Geometry check sheet. Reference: drawing and pictorial views, mm from the part's lowest x, y, z. A direction names the side the tool comes from. Coordinates: 2 decimals unless noted, no trailing zeros. Write each loop counter-clockwise with the first axis right and the second up, starting at its lowest first coordinate (ties: lowest second). Pieces come first, ordered by that corner, then holes. Notation, with made-up numbers: M 48.25,55 L 83.25,55 A23 ccw 83.25,91 Z; hole C 74.5,53 d7. An arc over 180 degrees is marked long. One line per item, written item: value.
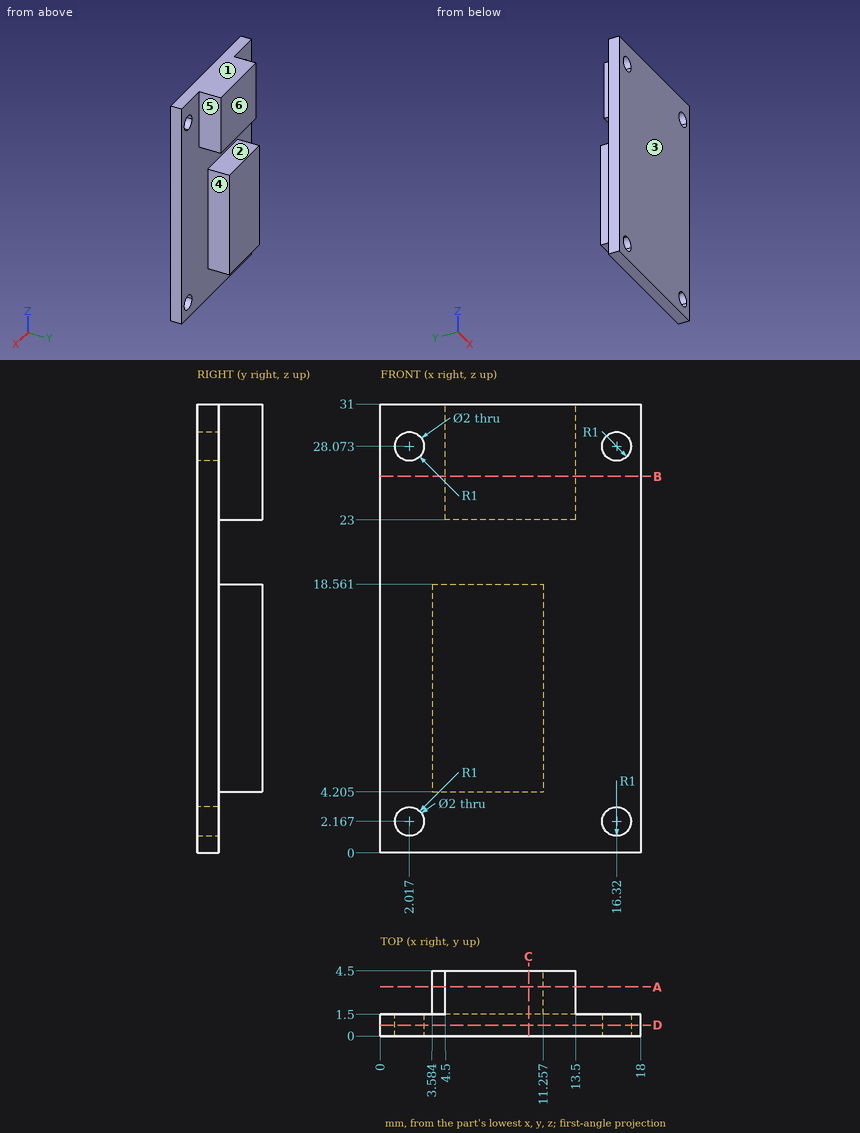
Item 1: Scan lines: line 1 (Z direction, x = 9.25, y = 4.15) (1 decimal); line 2 (Z direction, x = 12.5, y = 2.8); line 3 (Y direction, x = 5.25, z = 3). Record each from-to range of solid material in increasing order.
The answers:
line 1: z = 4.2 to 18.6, 23 to 31
line 2: z = 23 to 31
line 3: y = 0 to 1.5
Item 2: Cross-section at D-D, the plane y = 0.75. Enter the section's corners in (x, z).
The answers:
outline: M 0,0 L 18,0 L 18,31 L 0,31 Z; hole C 2.02,2.17 d2; hole C 2.02,28.07 d2; hole C 16.32,2.17 d2; hole C 16.32,28.07 d2
Item 3: Go/stop test with flat-tipped pins: P1, Ø0.9, axis at x = 8, y = 3, coming from the -Z side (1 decimal); P2, Ø1.2, axis at x = 2.02, z = 2.17, coming from the -Y side; P3, Ø1.5, axis at y = 3, z = 14.5, coming from the +X side. Record where each tip stops, or that it passes through.
The answers:
P1: stops at z = 4.2
P2: passes through
P3: stops at x = 11.26
Item 4: Cross-section at C-C, the plane x = 10.25. Enter the section's corners in (y, z) (1 decimal).
The answers:
outline: M 0,0 L 1.5,0 L 1.5,4.2 L 4.5,4.2 L 4.5,18.6 L 1.5,18.6 L 1.5,23 L 4.5,23 L 4.5,31 L 0,31 Z
Item 5: Cross-section at A-A, the plane y = 3.4. Enter the section's corners in (x, z) (1 decimal), and give its area (3 significant figures).
The answers:
outline: M 3.6,4.2 L 11.3,4.2 L 11.3,18.6 L 3.6,18.6 Z; M 4.5,23 L 13.5,23 L 13.5,31 L 4.5,31 Z
area: 182 mm²
Item 6: Access from +Z, -Z, +X, -X, +Y, -Y to the whole of each face (thin tool, end or side, straight path). Record for the marked faces 4, 5 and 6.
The answers:
face 4: -Z, +X, +Y
face 5: +Z, -Z, +X, +Y
face 6: +Z, -Z, +X, -X, +Y
Item 7: Cross-section at B-B, the plane z = 26. Enter the section's corners in (x, y), and give its area (3 significant figures).
The answers:
outline: M 0,0 L 18,0 L 18,1.5 L 13.5,1.5 L 13.5,4.5 L 4.5,4.5 L 4.5,1.5 L 0,1.5 Z
area: 54.0 mm²
Item 8: Draft check along Z on the marked faces 1, 2 and 3. Enter one of: released by +Z, released by -Z, zero draft, split by the parting line, or undercut.
The answers:
face 1: released by +Z
face 2: undercut
face 3: zero draft
